Read the model definition and answer for the solid it produces. Units are mm, in the model's axes. Face numbers are marked on the shaded views. A direction names the side the tool comes from. Coordinates: 2 decimals unless noted, no trailing zeros. Order: outer loops, then holes, each group sorted by start corner. A loop starts at its lowest first (then second) coordinate and runs counter-clockwise, first axis right, second up. Notation, with made-up numbers: (37, 64) -> (61, 64) arc R7 ccw to (61, 68) -> close; hole circle Ø5 at (51.5, 22). An arc over 180 degrees is marked (long way). Answer in a Markdown table with one row per item.
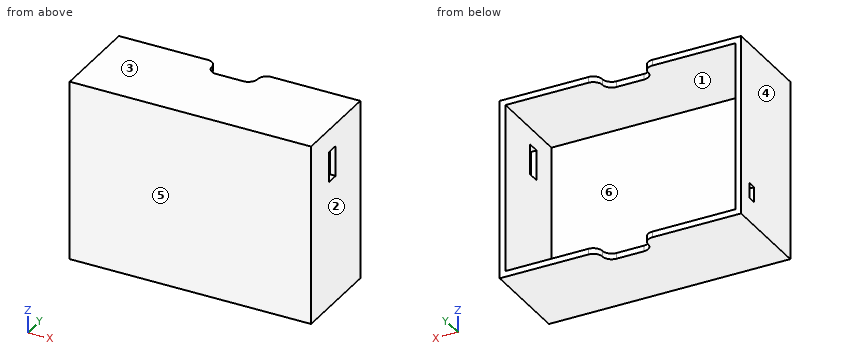
from build123d import *

# Parameters (mm, degrees)
SKETCH1_W           = 100.584
SKETCH1_H           = 75.184
BOSS_EXTRUDE1_DEPTH = 2.54
SKETCH2_W           = 100.584
SKETCH2_H           = 75.184
SKETCH2_W_2         = 95.758
SKETCH2_H_2         = 70.358
BOSS_EXTRUDE2_DEPTH = 35.56
SKETCH3_W           = 19.05
SKETCH3_H           = 7.62
CUT_EXTRUDE1_DEPTH  = 132.230274373
FILLET1_R           = 3.81
SKETCH4_W           = 6.35
SKETCH4_H           = 3.81
CUT_EXTRUDE2_DEPTH  = 6.35
SKETCH5_W           = 12.7
SKETCH5_H           = 5.08
CUT_EXTRUDE3_DEPTH  = 6.35


with BuildPart() as part:
    # Sketch1 → Boss-Extrude1 (new body)
    with BuildSketch(Plane(origin=(0, 0, 0), x_dir=(1, 0, 0), z_dir=(0, 1, 0))):
        with Locations((50.292, 37.592)):
            Rectangle(SKETCH1_W, SKETCH1_H)
    extrude(amount=BOSS_EXTRUDE1_DEPTH)

    # Sketch2 → Boss-Extrude2 (add)
    with BuildSketch(Plane(origin=(0, 2.54, 0), x_dir=(1, 0, 0), z_dir=(0, 1, 0))):
        with Locations((50.292, 37.592)):
            Rectangle(SKETCH2_W, SKETCH2_H)
        with Locations((50.292, 37.592)):
            Rectangle(SKETCH2_W_2, SKETCH2_H_2, mode=Mode.SUBTRACT)
    extrude(amount=BOSS_EXTRUDE2_DEPTH)

    # Sketch3 → Cut-Extrude1 (cut, through all)
    with BuildSketch(Plane(origin=(0, 0, -75.184), x_dir=(-1, 0, 0), z_dir=(0, 0, -1))):
        with Locations((-50.292, 34.29)):
            Rectangle(SKETCH3_W, SKETCH3_H)
    extrude(amount=-CUT_EXTRUDE1_DEPTH, mode=Mode.SUBTRACT)

    # Fillet1
    fillet1_edges = [part.edges().sort_by_distance(p)[0] for p in [
        (40.767, 30.48, -1.2065),
        (59.817, 30.48, -1.2065),
        (59.817, 30.48, -73.9775),
        (40.767, 30.48, -73.9775),
    ]]
    fillet(fillet1_edges, radius=FILLET1_R)
    fillet1_2_edges = [part.edges().sort_by_distance(p)[0] for p in [
        (40.767, 38.1, -1.2065),
        (59.817, 38.1, -1.2065),
        (59.817, 38.1, -73.9775),
        (40.767, 38.1, -73.9775),
    ]]
    fillet(fillet1_2_edges, radius=FILLET1_R - 0.0001)  # a hair under: the kernel refuses the full size

    # Sketch4 → Cut-Extrude2 (cut)
    with BuildSketch(Plane.ZY):
        with Locations((-62.103, 29.845254)):
            Rectangle(SKETCH4_W, SKETCH4_H)
    extrude(amount=-CUT_EXTRUDE2_DEPTH, mode=Mode.SUBTRACT)

    # Sketch5 → Cut-Extrude3 (cut)
    with BuildSketch(Plane(origin=(100.584, 0, 0), x_dir=(0, 0, -1), z_dir=(1, 0, 0))):
        with Locations((15.748, 16.510254)):
            Rectangle(SKETCH5_W, SKETCH5_H)
    extrude(amount=-CUT_EXTRUDE3_DEPTH, mode=Mode.SUBTRACT)


solid = part.part
Q1. The part is cut by section D-D (y = 36.5). Write down the section's boundary in (x, z).
Outcome:
| item | result |
|---|---|
| outline | (0, -75.18) -> (40.06, -75.18) -> (40.06, -72.77) -> (2.41, -72.77) -> (2.41, -2.41) -> (40.06, -2.41) -> (40.06, 0) -> (0, 0) -> close; (60.52, -75.18) -> (100.58, -75.18) -> (100.58, 0) -> (60.52, 0) -> (60.52, -2.41) -> (98.17, -2.41) -> (98.17, -72.77) -> (60.52, -72.77) -> close |
Q2. The part is cut by section B-B (y = 9). Write down the section's boundary in (x, z).
Outcome:
| item | result |
|---|---|
| outline | (0, -75.18) -> (100.58, -75.18) -> (100.58, 0) -> (0, 0) -> close; hole (2.41, -72.77) -> (98.17, -72.77) -> (98.17, -2.41) -> (2.41, -2.41) -> close |
Q3. The part is cut by section A-A (z = -18.5). Write down the section's boundary in (x, y).
Outcome:
| item | result |
|---|---|
| outline | (0, 0) -> (100.58, 0) -> (100.58, 13.97) -> (98.17, 13.97) -> (98.17, 2.54) -> (2.41, 2.54) -> (2.41, 38.1) -> (0, 38.1) -> close; (98.17, 19.05) -> (100.58, 19.05) -> (100.58, 38.1) -> (98.17, 38.1) -> close |
Q4. Consider line 1 (X direction, y = 9, z = -27); line 2 (Z direction, x = 87, y = 33); line 3 (Y direction, x = 39, z = -12.5). Determine where each line is inside the solid, lowest interval first.
Outcome:
| item | result |
|---|---|
| line 1 | 0 to 2.41, 98.17 to 100.58 |
| line 2 | -75.18 to -72.77, -2.41 to 0 |
| line 3 | 0 to 2.54 |
Q5. For the marked faces 5 and 6, determine the directions among +Z, -Z, +X, -X, +Y, -Y from which every point of the face is accessible in a straight line to the end or side of a thin tool.
Outcome:
| item | result |
|---|---|
| face 5 | +Z, -Z, +X, -X, -Y |
| face 6 | +Y |
Q6. For a pull along X with two mould halves and no side action, classify the marked faces 1, 2, 3 and 4 as pulls with the +X half, pulls with the -X half, needs draft (parallel to the pull), parting line crosses it, or undercut.
Outcome:
| item | result |
|---|---|
| face 1 | undercut |
| face 2 | pulls with the +X half |
| face 3 | needs draft |
| face 4 | pulls with the -X half |
Q7. The part is cut by section C-C (x = 20). Write down the section's boundary in (y, z), then the cut area to 3 significant figures.
Outcome:
| item | result |
|---|---|
| outline | (0, -75.18) -> (38.1, -75.18) -> (38.1, -72.77) -> (2.54, -72.77) -> (2.54, -2.41) -> (38.1, -2.41) -> (38.1, 0) -> (0, 0) -> close |
| area | 363 mm² |
Q8. Given pin 1 (0.7 mm diameter, centred on x = 49, z = -74, fed in from +Y); pin 2 (10 mm diameter, centred on x = 58, z = -38.5, fed in from +Y), each flat-ended and moving along its own axis, determine where each tip first touches the part or whether it passes through.
Outcome:
| item | result |
|---|---|
| pin 1 | y = 30.48 |
| pin 2 | y = 2.54 |
